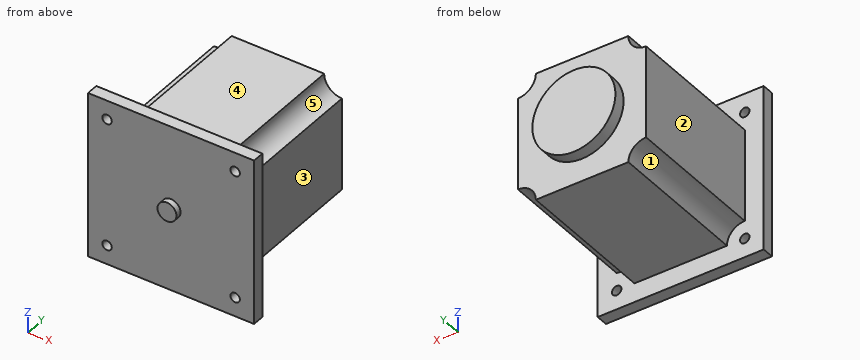
```python
from build123d import *

# Parameters (mm, degrees)
SKETCH_1_W      = 140
SKETCH_1_H      = 140
SKETCH_1_R      = 4
EXTRUDE_1_DEPTH = 10
EXTRUDE_2_DEPTH = 120
SKETCH_3_R      = 35
EXTRUDE_3_DEPTH = 10
SKETCH_4_R      = 8
EXTRUDE_4_DEPTH = 5


with BuildPart() as part:
    # 草图1 → 凸台-拉伸1 (new body)
    with BuildSketch(Plane(origin=(0, 0, 0), x_dir=(1, 0, 0), z_dir=(0, 1, 0))):
        Rectangle(SKETCH_1_W, SKETCH_1_H)
        with Locations((54, 54)):
            Circle(SKETCH_1_R, mode=Mode.SUBTRACT)
        with Locations((54, -54)):
            Circle(SKETCH_1_R, mode=Mode.SUBTRACT)
        with Locations((-54, -54)):
            Circle(SKETCH_1_R, mode=Mode.SUBTRACT)
        with Locations((-54, 54)):
            Circle(SKETCH_1_R, mode=Mode.SUBTRACT)
    extrude(amount=EXTRUDE_1_DEPTH)

    # 草图2 → 凸台-拉伸2 (add)
    with BuildSketch(Plane(origin=(0, 10, 0), x_dir=(1, 0, 0), z_dir=(0, 1, 0))):
        with BuildLine():
            Line((39, 54), (-39, 54))
            ThreePointArc((-39, 54), (-43.393398282, 43.393398282), (-54, 39))
            Line((-54, 39), (-54, -39))
            ThreePointArc((-54, -39), (-43.393398282, -43.393398282), (-39, -54))
            Line((-39, -54), (39, -54))
            ThreePointArc((39, -54), (43.393398282, -43.393398282), (54, -39))
            Line((54, -39), (54, 39))
            ThreePointArc((54, 39), (43.393398282, 43.393398282), (39, 54))
        make_face()
    extrude(amount=EXTRUDE_2_DEPTH)

    # 草图3 → 凸台-拉伸3 (add)
    with BuildSketch(Plane(origin=(0, 130, 0), x_dir=(1, 0, 0), z_dir=(0, 1, 0))):
        Circle(SKETCH_3_R)
    extrude(amount=EXTRUDE_3_DEPTH)

    # 草图4 → 凸台-拉伸4 (add)
    with BuildSketch(Plane.XZ):
        Circle(SKETCH_4_R)
    extrude(amount=EXTRUDE_4_DEPTH)


solid = part.part
```
Work out the finished part from the listing and answer in its coordinate system (mm). Face numbers are marked on the shaded views. A direction names the side the tool comes from. Give positions to 0.01 mm unless a question says otherwise; leave off trailing zeros. Write each loop counter-clockwise with the first axis right and the second up, starting at its lowest first coordinate (ties: lowest second). Pieces come first, ordered by that corner, then holes.
(1) The part is cut by section C-C on y = 14.5. Write down the section's boundary in (x, z).
Final values:
outline: (-54, -39) arc R15 cw to (-39, -54) - (39, -54) arc R15 cw to (54, -39) - (54, 39) arc R15 cw to (39, 54) - (-39, 54) arc R15 cw to (-54, 39) - close
(2) Which of the six approach directions +Z, -Z, +X, -X, +Y, -Y give full straight-line access (tool end or side, diameter ignored) to the marked faces 1, 2, 3, 4 and 5?
Final values:
face 1: -Z, -X, +Y
face 2: +Z, -Z, -X, +Y
face 3: +Z, -Z, +X, +Y
face 4: +Z, +X, -X, +Y
face 5: +Z, +X, +Y
(3) Straight lines are drawn through the part: line 1 (X direction, y = 4, z = 54); line 2 (X direction, y = 6, z = -53). For each, find the intervals that lie inside material, in ascending order.
Final values:
line 1: x = -70 to -58, -50 to 50, 58 to 70
line 2: x = -70 to -57.87, -50.13 to 50.13, 57.87 to 70
(4) The part is cut by section A-A on x = 0. Write down the section's boundary in (y, z).
Final values:
outline: (-5, -8) - (0, -8) - (0, -70) - (10, -70) - (10, -54) - (130, -54) - (130, -35) - (140, -35) - (140, 35) - (130, 35) - (130, 54) - (10, 54) - (10, 70) - (0, 70) - (0, 8) - (-5, 8) - close
(5) The part is cut by section B-B on z = 0. Write down the section's boundary in (x, y).
Final values:
outline: (-70, 0) - (-8, 0) - (-8, -5) - (8, -5) - (8, 0) - (70, 0) - (70, 10) - (54, 10) - (54, 130) - (35, 130) - (35, 140) - (-35, 140) - (-35, 130) - (-54, 130) - (-54, 10) - (-70, 10) - close
(6) Flat-ended cylindrical pins translate along their axes: pin 1 Ø4 at (x, y) = (-50, 83) entering from -Z; pin 2 Ø2 at (y, z) = (79, -18) entering from -X; pin 3 Ø6.5 at (x, z) = (-54, -54) entering from +Y (1 decimal); pin 4 Ø23.5 at (x, y) = (6.5, 97) entering from +Z. Find the tip coordinate at first contact, or state that the pin passes through.
Final values:
pin 1: stops at z = -40.25
pin 2: stops at x = -54
pin 3: passes through
pin 4: stops at z = 54
(7) The part is cut by section D-D on z = -29. Write down the section's boundary in (x, y), plus the area to 3 significant figures.
Final values:
outline: (-70, 0) - (70, 0) - (70, 10) - (54, 10) - (54, 130) - (19.6, 130) - (19.6, 140) - (-19.6, 140) - (-19.6, 130) - (-54, 130) - (-54, 10) - (-70, 10) - close
area: 14,800 mm2
